Autodesk Inventor part; units mm, degrees
ref_plane "YZ Plane" through (0, 0, 0) normal (1, 0, 0) x (0, 1, 0)
ref_plane "XZ Plane" through (0, 0, 0) normal (0, 1, 0) x (-1, 0, 0)
ref_plane "XY Plane" through (0, 0, 0) normal (0, 0, 1) x (1, 0, 0)
sketch "Skizze1" plane through (0, 0, 0) normal (0, 0, 1) x (1, 0, 0)
  line L0 (-22.5, 10) -> (22.5, 10)
  line L1 (22.5, 10) -> (22.5, -10)
  line L2 (22.5, -10) -> (-22.5, -10)
  line L3 (-22.5, -10) -> (-22.5, 10)
  line L4 (0, -14) -> (0, 14)
  line L5 (-31.5, 0) -> (31.5, 0)
  circle A0 centre (-11.25, 0) radius 8
  circle A1 centre (11.25, 0) radius 8
  circle A2 centre (-21.25, 8.75) radius 0.75
  circle A3 centre (21.25, 8.75) radius 0.75
  circle A4 centre (-21.25, -8.75) radius 0.75
  circle A5 centre (21.25, -8.75) radius 0.75
  circle A6 centre (-11.25, 0) radius 7
  circle A7 centre (11.25, 0) radius 7
  point P0 (0, 0)
  dimension "d0" = 20
  dimension "d1" = 45
  dimension "d2" = 16
  dimension "d3" = 11.25
  dimension "d4" = 1.5
  dimension "d5" = 1.25
  dimension "d6" = 1.25
  dimension "d11" = 1
  dimension "d12" = 1
extrude "Extrusion1" add sketch "Skizze1" against normal blind 4
extrude "Extrusion3" add sketch "Skizze1" along normal blind 12 contours A0 L5 A6 | L5 A6 A0 | A1 L5 A7 | L5 A7 A1
extrude "Extrusion4" add sketch "Skizze1" along normal blind 11.5 contours A6 L5 | L5 A6 | A7 L5 | L5 A7
properties part number "Ultraschallsensor"
Work out the finished part from the listing and answer in its coordinate system (mm). A direction names the side the tool comes from. Give positions to 0.01 mm unless a question says otherwise; leave off trailing zeros. Order: outer loops, then holes, each group sorted by start corner. A loop starts at its lowest first (then second) coordinate and runs counter-clockwise, first axis right, second up. Notation, with made-up numbers: (14.25, 16) -> (42.25, 16) arc R19 ccw to (42.25, 43) -> close; hole circle Ø8 at (53, 29). An arc over 180 degrees is marked (long way). Answer as a JSON object with one key per item and string values. Group by question number.
1. Section D-D on z = 8.5 is taken. Determine the outline of the cut face in (x, y).
2. Section C-C on x = -11.25 is taken. Determine the outline of the cut face in (y, z).
3. Consider line 1 along Y through (x, z) = (21.25, -1.4); line 2 along Y through (x, z) = (11.25, 11.7); line 3 along X through (y, z) = (0, 11.6). Determine where each line is inside the solid, lowest interval first. Write a range as [from, to].
4. Flat-ended cylindrical pins translate along their axes: pin 1 Ø4 at (x, z) = (9, 10) entering from -Y; pin 2 Ø8 at (x, z) = (-12.5, 9) entering from +Y; pin 3 Ø3 at (y, z) = (1.5, 4) entering from -X; pin 4 Ø0.9 at (x, y) = (-21.25, -8.75) entering from +Z (1 decimal). Find the tip coordinate at first contact, or state that the pin passes through.
5. A tool of negligible diameter and unlimited length cuts with its end or side. For faces 1 (the flat face through (-11, 0, 11.5)), 2 (the flat face through (0, -10, -2)), from which of +Z, -Z, +X, -X, +Y, -Y can it reach the whole face along a straight path? Write none if from no direction.
6. Section A-A on x = -21.25 is taken. Determine the outline of the cut face in (y, z), plus the area to 3 significant figures.
7. Section B-B on y = 8.75 is taken. Determine the outline of the cut face in (x, z), plus the area to 3 significant figures.
Result sheet:
{
 "1": {"outline": "circle Ø16 at (-11.25, 0); circle Ø16 at (11.25, 0)"},
 "2": {"outline": "(-10, -4) -> (10, -4) -> (10, 0) -> (8, 0) -> (8, 12) -> (7, 12) -> (7, 11.5) -> (-7, 11.5) -> (-7, 12) -> (-8, 12) -> (-8, 0) -> (-10, 0) -> close"},
 "3": {"line 1": "y = [-10, -9.5], [-8, 8], [9.5, 10]", "line 2": "y = [-8, -7], [7, 8]", "line 3": "x = [-19.25, -18.25], [-4.25, -3.25], [3.25, 4.25], [18.25, 19.25]"},
 "4": {"pin 1": "stops at y = -8", "pin 2": "stops at y = 8", "pin 3": "stops at x = -19.25", "pin 4": "passes through"},
 "5": {"face 1": "+Z", "face 2": "+Z, -Z, +X, -X, -Y"},
 "6": {"outline": "(-10, -4) -> (-9.5, -4) -> (-9.5, 0) -> (-10, 0) -> close; (-8, -4) -> (8, -4) -> (8, 0) -> (-8, 0) -> close; (9.5, -4) -> (10, -4) -> (10, 0) -> (9.5, 0) -> close", "area": "68.0 mm^2"},
 "7": {"outline": "(-22.5, -4) -> (-22, -4) -> (-22, 0) -> (-22.5, 0) -> close; (-20.5, -4) -> (20.5, -4) -> (20.5, 0) -> (-20.5, 0) -> close; (22, -4) -> (22.5, -4) -> (22.5, 0) -> (22, 0) -> close", "area": "168 mm^2"}
}
